Part model, mm, in its own coordinate system. A direction names the side the tool comes from. Round coordinates to 2 decimals unless told otherwise and drop trailing zeros. Order: outer loops, then holes, each group sorted by start corner. A loop starts at its lowest first (then second) coordinate and runs counter-clockwise, first axis right, second up. Notation, with made-up numbers: (14.25, -17.5) - (41.25, -17.5) arc R9 cw to (41.25, -10.5) - close; hole circle Ø6 at (-32, 89). An arc over 180 degrees is marked (long way). Answer as a JSON object with one key per item and string values.
```python
from build123d import *

# Parameters (mm, degrees)
SKETCH1_W                = 23
SKETCH1_H                = 12
BOSS_EXTRUDE1_DEPTH      = 6.6
BOSS_EXTRUDE2_DEPTH      = 5
BOSS_EXTRUDE2_DEPTH_BACK = 28
SKETCH2_W                = 12
SKETCH2_H                = 2
CUT_EXTRUDE1_DEPTH       = 5
SHELL3_OUTLINE_W         = 21
SHELL3_OUTLINE_H         = 10
SHELL3_DEPTH             = 5.6
SHELL3_2_DEPTH           = 1
SKETCH5_W                = 1
SKETCH5_H                = 10
BOSS_EXTRUDE4_DEPTH      = 1
SKETCH5_3_W              = 1
SKETCH5_3_H              = 10
BOSS_EXTRUDE5_DEPTH      = 1
BOSS_EXTRUDE6_DEPTH      = 4.4
CUT_EXTRUDE2_DEPTH       = 19.756598839
BOSS_EXTRUDE7_START      = -1
BOSS_EXTRUDE7_DEPTH      = 1
SKETCH21_R               = 2.5
SKETCH21_R_2             = 0.5
CUT_EXTRUDE3_DEPTH       = 21.718349355
SKETCH22_R               = 5.5
SKETCH22_R_2             = 0.8
CUT_EXTRUDE4_DEPTH       = 19.42851052
SKETCH23_R               = 0.8
SKETCH23_R_2             = 0.3
BOSS_EXTRUDE9_DEPTH      = 2.5
SKETCH25_R               = 3.5
SKETCH25_R_2             = 2.5
BOSS_EXTRUDE10_DEPTH     = 2


# Read off the part's stored shape, not the designer's step: Shell3
with BuildPart() as part:
    # Sketch1 → Boss-Extrude1 (new body)
    with BuildSketch(Plane(origin=(0, 0, 0), x_dir=(1, 0, 0), z_dir=(0, 1, 0))):
        Rectangle(SKETCH1_W, SKETCH1_H)
    extrude(amount=BOSS_EXTRUDE1_DEPTH)

    # Sketch2 → Boss-Extrude2 (add, two sides: drawn at the far end of the back side and taken through both)
    with BuildSketch(Plane(origin=(11.5, 0, 0), x_dir=(0, 0, -1), z_dir=(1, 0, 0)).offset(-BOSS_EXTRUDE2_DEPTH_BACK)):
        with Locations((0, 1)):
            Rectangle(SKETCH2_W, SKETCH2_H)
    extrude(amount=BOSS_EXTRUDE2_DEPTH + BOSS_EXTRUDE2_DEPTH_BACK)

    # Sketch3 → Cut-Extrude1 (cut)
    with BuildSketch(Plane(origin=(0, 2, 0), x_dir=(1, 0, 0), z_dir=(0, 1, 0))):
        with BuildLine():
            Line((16.5, 0.65), (15.5, 0.65))
            ThreePointArc((15.5, 0.65), (13.750113293, -0.026490152), (15.519570239, -0.65))
            Line((15.519570239, -0.65), (16.5, -0.65))
            Line((16.5, -0.65), (16.5, 0.65))
        make_face()
        with BuildLine():
            Line((-16.5, -0.65), (-16.5, 0.65))
            Line((-16.5, 0.65), (-15.5, 0.65))
            ThreePointArc((-15.5, 0.65), (-13.750113293, -0.026490152), (-15.519570239, -0.65))
            Line((-15.519570239, -0.65), (-16.5, -0.65))
        make_face()
    extrude(amount=-CUT_EXTRUDE1_DEPTH, mode=Mode.SUBTRACT)

    # Shell3 outline → Shell3 (cut)
    with BuildSketch(Plane(origin=(0, 0, 0), x_dir=(1, 0, 0), z_dir=(0, 1, 0))):
        Rectangle(SHELL3_OUTLINE_W, SHELL3_OUTLINE_H)
    extrude(amount=SHELL3_DEPTH, mode=Mode.SUBTRACT)

    # Shell3 2 outline → Shell3 2 (cut)
    with BuildSketch(Plane(origin=(0, 0, 0), x_dir=(1, 0, 0), z_dir=(0, 1, 0))):
        with BuildLine():
            ThreePointArc((-15.5, 1.842611794), (-12.75, -0.011437828), (-15.5, -1.86548745))
            Line((-15.5, -1.86548745), (-15.5, -5))
            Line((-15.5, -5), (-10.5, -5))
            Line((-10.5, -5), (-10.5, 5))
            Line((-10.5, 5), (-15.5, 5))
            Line((-15.5, 5), (-15.5, 1.842611794))
        make_face()
        with BuildLine():
            Line((10.5, 5), (10.5, -5))
            Line((10.5, -5), (15.5, -5))
            Line((15.5, -5), (15.5, -1.86548745))
            ThreePointArc((15.5, -1.86548745), (12.75, -0.011437828), (15.5, 1.842611794))
            Line((15.5, 1.842611794), (15.5, 5))
            Line((15.5, 5), (10.5, 5))
        make_face()
    extrude(amount=SHELL3_2_DEPTH, mode=Mode.SUBTRACT)

    # Sketch5 → Boss-Extrude4 (add)
    with BuildSketch(Plane.XZ.offset(-1)):
        with Locations((11, 0)):
            Rectangle(SKETCH5_W, SKETCH5_H)
    extrude(amount=BOSS_EXTRUDE4_DEPTH)

    # Sketch5<3> → Boss-Extrude5 (add)
    with BuildSketch(Plane.XZ.offset(-1)):
        with Locations((11, 0)):
            Rectangle(SKETCH5_3_W, SKETCH5_3_H)
        with Locations((-11, 0)):
            Rectangle(SKETCH5_3_W, SKETCH5_3_H)
    extrude(amount=BOSS_EXTRUDE5_DEPTH)

    # Sketch7 → Boss-Extrude6 (add)
    with BuildSketch(Plane(origin=(0, 6.6, 0), x_dir=(1, 0, 0), z_dir=(0, 1, 0))):
        with BuildLine():
            ThreePointArc((-0.1075, 2.630768661), (-11.5, 0), (-0.1075, -2.630768661))
            ThreePointArc((-0.1075, -2.630768661), (3.2, 0), (-0.1075, 2.630768661))
        make_face()
        with BuildLine():
            ThreePointArc((-0.3825, -2.01524037), (2.7, 0), (-0.3825, 2.01524037))
            ThreePointArc((-0.3825, 2.01524037), (-11, 0), (-0.3825, -2.01524037))
        make_face(mode=Mode.SUBTRACT)
    extrude(amount=BOSS_EXTRUDE6_DEPTH)

    # Sketch19 → Cut-Extrude2 (cut, through all)
    with BuildSketch(Plane(origin=(0, 6.6, 0), x_dir=(1, 0, 0), z_dir=(0, 1, 0))):
        with BuildLine():
            ThreePointArc((-0.409482759, 2.082458695), (-11, 0), (-0.409482759, -2.082458695))
            ThreePointArc((-0.409482759, -2.082458695), (2.5, 0), (-0.409482759, 2.082458695))
        make_face()
    extrude(amount=-CUT_EXTRUDE2_DEPTH, mode=Mode.SUBTRACT)

    # Sketch20 → Boss-Extrude7 (add)
    with BuildSketch(Plane(origin=(0, 11, 0), x_dir=(1, 0, 0), z_dir=(0, 1, 0)).offset(BOSS_EXTRUDE7_START)):
        with BuildLine():
            ThreePointArc((-0.125, 2.666341126), (-11.5, 0), (-0.125, -2.666341126))
            ThreePointArc((-0.125, -2.666341126), (3, 0), (-0.125, 2.666341126))
        make_face()
    extrude(amount=BOSS_EXTRUDE7_DEPTH)

    # Sketch21 → Cut-Extrude3 (cut, through all)
    with BuildSketch(Plane(origin=(0, 11, 0), x_dir=(1, 0, 0), z_dir=(0, 1, 0))):
        with Locations(Location((-5.5, 0, 0), (0, 0, 270))):
            Circle(SKETCH21_R)
        with Locations(Location((0.5, 0, 0), (0, 0, 270))):
            Circle(SKETCH21_R_2)
    extrude(amount=-CUT_EXTRUDE3_DEPTH, mode=Mode.SUBTRACT)

    # Sketch22 → Cut-Extrude4 (cut, through all)
    with BuildSketch(Plane.XZ.offset(-5.6)):
        with Locations((0.5, 0)):
            Circle(SKETCH22_R)
        with Locations((-10.2, 4.7)):
            Circle(SKETCH22_R_2)
        with Locations((-10.2, -4.7)):
            Circle(SKETCH22_R_2)
        with Locations((10.2, -4.7)):
            Circle(SKETCH22_R_2)
        with Locations((10.2, 4.7)):
            Circle(SKETCH22_R_2)
    extrude(amount=CUT_EXTRUDE4_DEPTH, mode=Mode.SUBTRACT)

    # Sketch23 → Boss-Extrude9 (add)
    # profile 1 of 4: a face of its own
    with BuildSketch(Plane.XZ.offset(-5.6)):
        with Locations((-10.2, 4.7)):
            Circle(SKETCH23_R)
        with Locations(Location((-10.2, 4.7, 0), (0, 0, 270))):
            Circle(SKETCH23_R_2, mode=Mode.SUBTRACT)
    # profile 2 of 4: a face of its own
    with BuildSketch(Plane.XZ.offset(-5.6)):
        with Locations((-10.2, -4.7)):
            Circle(SKETCH23_R)
        with Locations(Location((-10.2, -4.7, 0), (0, 0, 90))):
            Circle(SKETCH23_R_2, mode=Mode.SUBTRACT)
    # profile 3 of 4: a face of its own
    with BuildSketch(Plane.XZ.offset(-5.6)):
        with Locations((10.2, -4.7)):
            Circle(SKETCH23_R)
        with Locations(Location((10.2, -4.7, 0), (0, 0, 270))):
            Circle(SKETCH23_R_2, mode=Mode.SUBTRACT)
    # profile 4 of 4: a face of its own
    with BuildSketch(Plane.XZ.offset(-5.6)):
        with Locations((10.2, 4.7)):
            Circle(SKETCH23_R)
        with Locations(Location((10.2, 4.7, 0), (0, 0, 90))):
            Circle(SKETCH23_R_2, mode=Mode.SUBTRACT)
    extrude(amount=BOSS_EXTRUDE9_DEPTH)

    # Sketch25 → Boss-Extrude10 (add)
    with BuildSketch(Plane.XZ.offset(-10)):
        with Locations(Location((-5.5, 0, 0), (0, 0, 90))):
            Circle(SKETCH25_R)
        with Locations(Location((-5.5, 0, 0), (0, 0, 90))):
            Circle(SKETCH25_R_2, mode=Mode.SUBTRACT)
    extrude(amount=BOSS_EXTRUDE10_DEPTH)


solid = part.part
```
Item 1: Cut at C-C (y = 3.75). Write the cut outline in (x, z).
Taken from the geometry:
{"outline": "(-11.5, -6) - (11.5, -6) - (11.5, 6) - (-11.5, 6) - close; hole circle Ø0.6 at (-10.2, -4.7); hole (-10.5, -3.96) arc R0.8 cw to (-9.46, -5) - (-7.79, -5) arc R5.5 ccw to (-3.21, -5) - (-1.79, -5) arc R5.5 ccw to (2.79, -5) - (9.46, -5) arc R0.8 cw to (10.5, -3.96) - (10.5, 3.96) arc R0.8 cw to (9.46, 5) - (2.79, 5) arc R5.5 ccw to (-1.79, 5) - (-3.21, 5) arc R5.5 ccw to (-7.79, 5) - (-9.46, 5) arc R0.8 cw to (-10.5, 3.96) - (-10.5, 2.29) arc R5.5 ccw to (-10.5, -2.29) - close; hole circle Ø0.6 at (-10.2, 4.7); hole circle Ø0.6 at (10.2, -4.7); hole circle Ø0.6 at (10.2, 4.7)"}
Item 2: Cut at D-D (x = -12). Write the cut outline in (y, z), plus the area to 3 significant figures.
Taken from the geometry:
{"outline": "(0, -6) - (2, -6) - (2, 6) - (0, 6) - (0, 5) - (1, 5) - (1, -5) - (0, -5) - close", "area": "14.0 mm2"}
Item 3: Tool access for faces 5 (the flat face through (-10.5, 3, -3)), 6 (the flat face through (-16, 1, -0.65)), 7 (the flat face through (16, 1, -0.65)), 8 (the cylindrical face through (2.7, 8.28, 0.06)): list every direction of +Z, -Z, +X, -X, +Y, -Y with a clear straight run to the whole face (end or side of a thin tool).
Taken from the geometry:
{"face 5": "-Y", "face 6": "-X, +Y, -Y", "face 7": "+X, +Y, -Y", "face 8": "none"}
Item 4: Cut at A-A (y = 9.5). Write the cut outline in (x, z), plus the area to 3 significant figures.
Taken from the geometry:
{"outline": "circle Ø7 at (-5.5, 0); (-0.11, -2.63) arc R2.7 ccw (long way) to (-0.11, 2.63) arc R6 ccw (long way) to start; hole circle Ø5 at (-5.5, 0); hole (-0.38, -2.02) arc R2.2 ccw (long way) to (-0.38, 2.02) arc R5.5 ccw (long way) to start", "area": "39.1 mm2"}
Item 5: Cut at B-B (x = 14.75). Write the cut outline in (y, z).
Taken from the geometry:
{"outline": "(0, -6) - (2, -6) - (2, -0.99) - (0, -0.99) - (0, -1.99) - (1, -1.99) - (1, -5) - (0, -5) - close; (0, 1.01) - (2, 1.01) - (2, 6) - (0, 6) - (0, 5) - (1, 5) - (1, 2.01) - (0, 2.01) - close"}
Item 6: Drop flat-ended pins along their axis: P1, Ø3, axis at x = 5.5, z = -5, coming from the +Y side; P2, Ø2, axis at x = -8, z = -3, coming from the -Y side; P3, Ø0.5, axis at x = 10, z = -5, coming from the -Y side. Give the stop position or say it passes through.
Taken from the geometry:
{"P1": "y = 6.6", "P2": "y = 8", "P3": "y = 3.1"}
Item 7: Probe L1, parallel to X at y = 8.6, z = 0; L2, parallel to X at y = 3.75, z = 4.75; L3, parallel to X at y = 4.75, z = 0. List the from-to ranges inside material, lowest first. Write a range as from..to.
Taken from the geometry:
{"L1": "-11.5..-11, -9..-8, -3..-2, 2.7..3.2", "L2": "-11.5..-10.5, -9.9..-9.4, 9.4..9.9, 10.5..11.5", "L3": "-11.5..-11, 10.5..11.5"}
Item 8: Two-plate mould, pull along Z, no slides. Class faces 1 (the cylindrical face through (-2.083, 9.014, -0.759)), 2 (the flat face through (-11.5, 4, 0)), 3 (the flat face through (15.5, 0.5, 3.5)), 4 (the flat face through (0, 3, -6)): pulls with the +Z half, pulls with the -Z half, needs draft (parallel to the pull), parting line crosses it, or undercut.
Taken from the geometry:
{"face 1": "undercut", "face 2": "needs draft", "face 3": "undercut", "face 4": "pulls with the -Z half"}
